Here's how the part is built. I have some questions about the finished solid (model axes, mm). Face numbers are marked on the shaded views. A direction names the side the tool comes from. Round coordinates to 2 decimals unless told otherwise and drop trailing zeros. Order: outer loops, then holes, each group sorted by start corner. A loop starts at its lowest first (then second) coordinate and runs counter-clockwise, first axis right, second up. Notation, with made-up numbers: (42.5, 32.25) - (52.5, 32.25) arc R7 ccw to (52.5, 43.25) - close; hole circle Ø7 at (49, 59.25). An arc over 180 degrees is marked (long way). One line per item, written item: value.
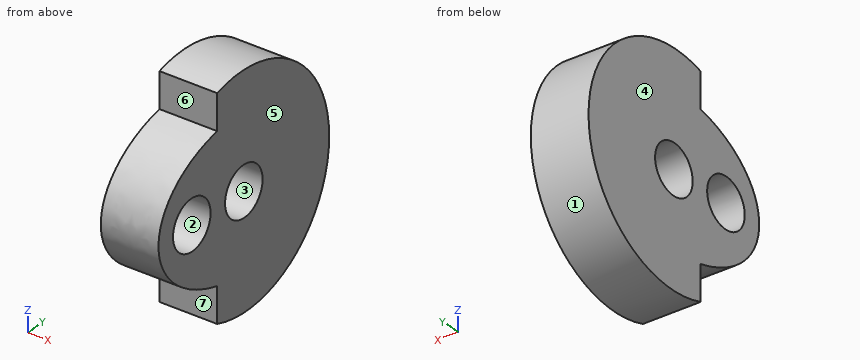
from build123d import *

# Parameters (mm, degrees)
BOSS_EXTRUDE1_DEPTH             = 13
M10_CLEARANCE_HOLE2_D           = 11
M10_CLEARANCE_HOLE2_ON_FACE_2_D = 11
M10_CLEARANCE_HOLE1_D           = 11


with BuildPart() as part:
    # Sketch1 → Boss-Extrude1 (new body)
    with BuildSketch(Plane(origin=(0, 0, 0), x_dir=(0, 0, -1), z_dir=(1, 0, 0))):
        with BuildLine():
            Line((-23.749988068, -7.8062838), (-15.929764022, -7.8062838))
            add(Edge.make_bspline(
                [(-15.929764022, -7.8062838), (0, -80.063704579), (15.929764022, -7.8062838)],
                knots=[5.029950938, 5.029950938, 5.029950938, 7.536419676, 7.536419676, 7.536419676], degree=2, weights=[1, 0.312251352, 1]))
            Line((15.929764022, -7.8062838), (23.749988068, -7.8062838))
            ThreePointArc((23.749988068, -7.8062838), (0, 25), (-23.749988068, -7.8062838))
        make_face()
    extrude(amount=BOSS_EXTRUDE1_DEPTH)

    # M10 Clearance Hole2 (through all)
    with Locations(Plane(origin=(0, 0, 0), x_dir=(0, 0, -1), z_dir=(-1, 0, 0))):
        with Locations((0, 0)):
            Hole(M10_CLEARANCE_HOLE2_D / 2)

    # M10 Clearance Hole2 on face 2 (through all)
    with Locations(Plane(origin=(13, 0, 0), x_dir=(0, 0, 1), z_dir=(1, 0, 0))):
        with Locations((0, 0)):
            Hole(M10_CLEARANCE_HOLE2_ON_FACE_2_D / 2)

    # M10 Clearance Hole1 (through all)
    with Locations(Plane(origin=(13, -15.25, 0), x_dir=(0, 0, 1), z_dir=(1, 0, 0))):
        with Locations((0, 0)):
            Hole(M10_CLEARANCE_HOLE1_D / 2)


solid = part.part
Q1. Which directions (+Z, -Z, +X, -X, +Y, -Y) give clear straight access to the entire face, cutting with the end or side of a thin tool? Please do the marked faces 5, 6 and 7.
Results list:
face 5: +Z, -Z, +X, +Y, -Y
face 6: +Z, +X, -X, -Y
face 7: -Z, +X, -X, -Y
Q2. We'd pull the mould along Z, two halves only. Please class the marked faces 1, 2, 3 and 4: released by +Z, released by -Z, zero draft, split by the parting line, or undercut.
Results list:
face 1: split by the parting line
face 2: undercut
face 3: undercut
face 4: zero draft
Q3. If we section it at D-D, the plane y = -7: Please give me the cut outline in (x, z).
Results list:
outline: (0, -24) - (13, -24) - (13, 24) - (0, 24) - close
Q4. If I drill on line 1 along Y through (x, z) = (10.5, -0.5) (3 decimals); line 2 along Y through (x, z) = (4.5, 1); line 3 along Z through (x, y) = (0.75, 4.5), over which ranges is the centre line in solid material (lowest first)?
Results list:
line 1: -24.989 to -20.727, -9.773 to -5.477, 5.477 to 24.995
line 2: -24.96 to -20.66, -9.84 to -5.41, 5.41 to 24.98
line 3: -24.59 to -3.16, 3.16 to 24.59
Q5. If we section it at A-A, the plane y = 0: Please give me the cut outline in (x, z), then the cut area to 3 significant figures.
Results list:
outline: (0, -25) - (13, -25) - (13, -5.5) - (0, -5.5) - close; (0, 5.5) - (13, 5.5) - (13, 25) - (0, 25) - close
area: 507 mm²
Q6. Will these pins go through, and if not, where does the flat tip stop? pin 1 (6 mm diameter, centred on x = 2.5, z = -19, fed in from +Y); pin 2 (2 mm diameter, centred on y = 14, z = -13.5, fed in from -X); pin 3 (4 mm diameter, centred on x = 8.5, y = 15.5, fed in from -Z); pin 4 (2 mm diameter, centred on x = 8, y = -17, fed in from -Z).
Results list:
pin 1: y = 19.21
pin 2: x = 0
pin 3: z = -21.04
pin 4: z = -12.88
Q7. If we section it at B-B, the plane z = 0: Give the number of separate pieces and of enclosed holes in the cut face, then the cut area to 3 significant figures.
Results list:
separate pieces: 3
enclosed holes: 0
area: 364 mm²
